Can you work these out from the model? Positions are in its coordinate system, mm. Face numbers are marked on the shaded views. Give positions to 0.01 mm unless a question says otherwise; leave off trailing zeros. Order: outer loops, then holes, each group sorted by start corner. A loop starts at its lowest first (then second) coordinate and runs counter-clockwise, first axis right, second up. Notation, with made-up numbers: M -22,-20.5 L 11,-20.5 A33 cw 11,13.5 Z; hole C -21,11.25 d5. An arc over 180 degrees is marked long. One line per question, with ' | ' between items. Start each with the question number.
1) Please list where these lines run through material, in increasing order: line 1 along X through (y, z) = (17.5, 3); line 2 along Y through (x, z) = (13.5, 196.5); line 3 along X through (y, z) = (-42.5, 140). Write a range as [from, to].
2) I'm going to push flat-ended pins straight in: pin 1 Ø12 at (x, z) = (-1, -162) entering from -Y; pin 2 Ø10 at (y, z) = (-42, 158) entering from -X; pin 3 Ø4 at (y, z) = (6.5, 227.5) entering from -X. Where does each tip first touch, or does it pass through?
3) If we section it at B-B, the plane z = -32: Please give me the cut outline in (x, y), plus the area to 3 significant figures.
4) If we section it at C-C, the plane x = 17: Please give me the cut outline in (y, z).
5) Thinking about a two-plate mould opening in Z: for the marked faces 1, 2 and 3, which applies, +Z half, -Z half, draft (parallel to the pull), parting line (faces both ways), or undercut?
6) If we section it at D-D, the plane z = -219: Please give me the cut outline in (x, y), plus the area to 3 significant figures.
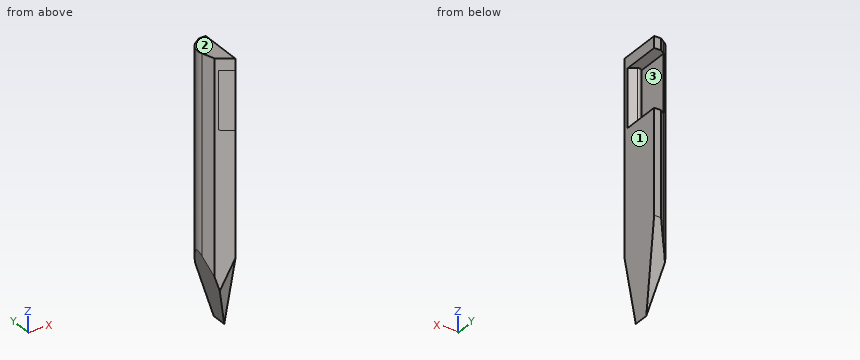
Autodesk Inventor part; units mm, degrees
ref_plane "YZ Plane" through (0, 0, 0) normal (1, 0, 0) x (0, 1, 0)
ref_plane "XZ Plane" through (0, 0, 0) normal (0, 1, 0) x (-1, 0, 0)
ref_plane "XY Plane" through (0, 0, 0) normal (0, 0, 1) x (1, 0, 0)
sketch "Sketch1" plane through (0, 0, 0) normal (0, 0, 1) x (1, 0, 0)
  line L0 (-25, -57.5) -> (25, -57.5)
  line L1 (25, -57.5) -> (25, 57.5)
  line L2 (25, 57.5) -> (-25, 57.5)
  line L3 (-25, 57.5) -> (-25, -57.5)
  line L4 (-25, -57.5) -> (25, 57.5) construction
  line L5 (25, -57.5) -> (-25, 57.5) construction
  point P0 (0, 0)
  dimension "d0" = 50
  dimension "d1" = 115
extrude "Extrusion1" add sketch "Sketch1" along normal mid plane 800
sketch "Sketch2" plane through (0, 0, 400) normal (0, 0, 1) x (1, 0, 0)
  line L0 (-25, -57.5) -> (25, -57.5)
  line L1 (25, -57.5) -> (25, 57.5) construction
  line L2 (25, 57.5) -> (-25, 57.5)
  line L3 (-25, 57.5) -> (-25, -57.5)
  line L4 (25, -57.5) -> (86.0387, -57.5) construction
  line L5 (-25, -57.5) -> (25, -57.5)
  line L6 (25, -57.5) -> (-11.8618, -31.6891)
  line L7 (25, -57.5) -> (70, -57.5) construction
  line L8 (-11.8618, -31.6891) -> (-22.6774, 1.5979)
  line L9 (-11.8618, -31.6891) -> (23.1382, -31.6891) construction
  arc A0 (-3.649, 50.0435) -> (-22.6774, 1.5979) centre (15.1106, 14.7153) ccw
  line L10 (-3.649, 50.0435) -> (7, 57.5)
  line L11 (-3.649, 50.0435) -> (9.351, 50.0435) construction
  line L12 (25, 57.5) -> (-25, 57.5)
  point P0 (0, 0)
  dimension "d5" = 45
  dimension "d6" = 145
  dimension "d7" = 35
  dimension "d8" = 108
  dimension "d9" = 40
  dimension "d10" = 13
  dimension "d11" = 35
  dimension "d12" = 18
extrude "Extrusion2" cut sketch "Sketch2" against normal through all
sketch "Sketch3" plane through (0, 0, 0) normal (1, 0, 0) x (0, 1, 0)
  line L0 (57.5, -400) -> (57.5, 400)
  line L1 (-57.5, 400) -> (57.5, 400)
  line L2 (-57.5, -400) -> (-57.5, 400)
  line L3 (57.5, -400) -> (-57.5, -400)
  line L4 (-57.5, -400) -> (-57.5, 400)
  line L5 (-57.5, -100) -> (12.5, -400)
  line L6 (57.5, -400) -> (-57.5, -400)
  point P0 (0, 0)
  dimension "d15" = 300
  dimension "d16" = 70
extrude "Extrusion3" cut sketch "Sketch3" along normal through all both and the other way through all contours L3 L2 L5
sketch "Sketch4" plane through (25, 57.5, 400) normal (1, 0, 0) x (0, 0, -1)
  line L0 (500, -115) -> (800, -45)
  line L1 (800, 0) -> (800, -45)
  line L2 (800, 0) -> (0, 0)
  line L3 (0, -115) -> (0, 0)
  line L4 (500, -115) -> (0, -115)
  line L5 (800, -45) -> (450, 0)
  point P0 (400, -57.5)
  dimension "d19" = 350
extrude "Extrusion4" cut sketch "Sketch4" along normal through all both and the other way through all contours L5 L2 L1
sketch "Sketch5" plane through (0, 0, 0) normal (0, 1, 0) x (-1, 0, 0)
  line L0 (-25, -100) -> (-25, -400)
  line L1 (24.8894, -382.7696) -> (24.8894, 400)
  line L2 (-25, -400) -> (24.8894, -400)
  line L3 (24.8894, -400) -> (24.8894, 400)
  line L4 (-25, 400) -> (-25, -400)
  line L5 (-7, 400) -> (3.649, 400)
  line L6 (24.8894, -100) -> (-55, -400)
  line L7 (-55, -400) -> (-25, -400)
  point P0 (0, 0)
  point P1 (-0.0553, 400)
  dimension "d22" = 30
  dimension "d23" = 300
extrude "Extrusion5" cut sketch "Sketch5" along normal through all both and the other way through all
sketch "Sketch6" plane through (7, 57.5, 400) normal (0, 1, 0) x (1, 0, 0)
  line L0 (18, 500) -> (18, 0)
  line L1 (18, 30) -> (-12, 30)
  line L2 (-12, 30) -> (-12, 180)
  line L3 (-12, 180) -> (18, 180)
  line L4 (18, 180) -> (18, 30)
  line L5 (18, 0) -> (0, 0)
  point P0 (-7, 400)
  dimension "d26" = 30
  dimension "d27" = 150
  dimension "d28" = 30
extrude "Extrusion6" cut sketch "Sketch6" against normal through all
sketch "Sketch7" plane through (-11.8618, -31.6891, -148.9211) normal (-0.5735764, -0.819152, 0) x (0.819152, -0.5735764, 0)
  line L0 (-40.8281, 518.9211) -> (8.3768, 518.9211)
  line L1 (-20.9613, 368.9211) -> (45, 368.9211)
  line L2 (8.3768, 518.9211) -> (45, 518.9211)
  line L3 (45, 518.9211) -> (45, 368.9211)
  line L4 (45, 368.9211) -> (8.3768, 368.9211)
  line L5 (8.3768, 368.9211) -> (8.3768, 518.9211)
  point P0 (-8.4594, 148.9211)
extrude "Extrusion7" add sketch "Sketch7" against normal blind 10
fillet "Fillet1" radius 8 1 edges at (0.7358, -28.3023, 295)
sketch "Sketch8" plane through (25, -57.5, 370) normal (0, 0, 1) x (1, 0, 0)
  line L0 (0, 0) -> (0, 12.2077)
  line L1 (0, 0) -> (5.7358, 8.1915)
  line L2 (0, 12.2077) -> (5.7358, 8.1915)
  point P0 (-25, 57.5)
extrude "Extrusion8" cut sketch "Sketch8" against normal through all
properties part number "bodyside"
Results found:
1) line 1: x = [-24.79, 25] | line 2: y = [-49.45, 57.5] | line 3: x = [3.58, 25]
2) pin 1: stops at y = -43.37 | pin 2: stops at x = -4.28 | pin 3: stops at x = -24.4
3) outline: M -22.68,1.6 L -11.86,-31.69 L 25,-57.5 L 25,57.5 L 7,57.5 L -3.65,50.04 A40 ccw Z | area: 4,250 mm²
4) outline: M -51.9,-124.01 L -20.8,-257.3 L 30.85,-257.3 L 57.5,-50 L 57.5,220 L -39.69,220 L -39.69,370 L 57.5,370 L 57.5,400 L -51.9,400 Z
5) face 1: draft | face 2: +Z half | face 3: undercut
6) outline: M 6.8,-29.73 L 25,-29.73 L 25,35.77 L 6.8,35.77 Z | area: 1,190 mm²
